from build123d import *

# Parameters (mm, degrees)
BOSS_EXTRU_1_DEPTH   = 3
ESQUISSE2_R          = 2.55
BOSS_EXTRU_2_DEPTH   = 3.2
CONG_1_R             = 1.8
D_GAGEMENT_M31_D     = 3.4
D_GAGEMENT_M31_DEPTH = 5
D_GAGEMENT_M31_TIP   = 1.021463052


with BuildPart() as part:
    # Esquisse1 → Boss.-Extru.1 (new body)
    with BuildSketch(Plane(origin=(0, 0, 0), x_dir=(1, 0, 0), z_dir=(0, 1, 0))):
        Polygon((3.117691454, 0), (1.558845727, 2.7), (-1.558845727, 2.7), (-3.117691454, 0), (-1.558845727, -2.7), (1.558845727, -2.7), align=None)
    extrude(amount=BOSS_EXTRU_1_DEPTH)

    # Esquisse2 → Boss.-Extru.2 (add)
    with BuildSketch(Plane(origin=(0, 3, 0), x_dir=(1, 0, 0), z_dir=(0, 1, 0))):
        with Locations(Location((0, 0, 0), (0, 0, 270))):
            Circle(ESQUISSE2_R)
    extrude(amount=BOSS_EXTRU_2_DEPTH)

    # Congé1
    cong_1_edges = [part.edges().sort_by_distance(p)[0] for p in [
        (0, 6.2, -2.55),
    ]]
    fillet(cong_1_edges, radius=CONG_1_R)

    # Dégagement M31
    with Locations(Plane(origin=(0, 0, 0), x_dir=(-1, 0, 0), z_dir=(0, -1, 0))):
        with Locations((0, 0)):
            Hole(D_GAGEMENT_M31_D / 2, depth=D_GAGEMENT_M31_DEPTH)
            with Locations((0, 0, -(D_GAGEMENT_M31_DEPTH + D_GAGEMENT_M31_TIP / 2))):  # 118° drill point
                Cone(0, D_GAGEMENT_M31_D / 2, D_GAGEMENT_M31_TIP, mode=Mode.SUBTRACT)


solid = part.part
Geometry check sheet. Reference: the model listing, model coordinates, mm. A direction names the side the tool comes from. Coordinates: 2 decimals unless noted, no trailing zeros. Loops run counter-clockwise (first coordinate to the right, second up) from the corner with the lowest first, then second, coordinate; pieces in that order, holes last. Notation, with made-up numbers: (43.5, -13.75) - (83.5, -13.75) arc R22 ccw to (83.5, -7.75) - close; hole circle Ø11 at (1, 45.25). An arc over 180 degrees is marked (long way). Use one line per item in the form item = value. Start each with the question number.
Item 1: Section check A-A, the plane y = 2.75. Enter the section's corners in (x, z).
Item 2: Mould release check, pull along Z, two halves, no side actions. Record for faces 1 (the face through (-0.37, 2.54, 1.66)), 2 (the face through (0, 1, 2.7)), 3 (the face through (0.064, 5.844, 0.288)), 4 (the face through (2.35, 1.48, -1.33)): +Z half, -Z half, draft (parallel to the pull), parting line (faces both ways), or undercut.
Item 3: Gauge pin test, flat ends, axial feed: pin 1 (1 mm diameter, centred on x = 1, z = -1.5, fed in from +Y); pin 2 (1 mm diameter, centred on y = 4.5, z = 1.5, fed in from -X); pin 3 (2 mm diameter, centred on x = 2, z = -2, fed in from +Y). Record the tip position at first contact, or that the pin passes through.
Item 4: Tool access check on faces 5 (the face through (-2.35, 1.48, 1.33)), 6 (the face through (0.77, 3.69, 2.43)). Record the directions out of +Z, -Z, +X, -X, +Y, -Y that give a thin tool (end or side, any length) a straight path to the whole face; none if there is none.
Item 5: Thickness scan on probe 1 along Z at (x, y) = (0, 1.5); probe 2 along Y at (x, z) = (-2.5, -0.65); probe 3 along Z at (x, y) = (1, 1.5). Record the ranges inside material, lowest first.
Computed:
q1.outline = (-3.12, 0) - (-1.56, -2.7) - (1.56, -2.7) - (3.12, 0) - (1.56, 2.7) - (-1.56, 2.7) - close; hole circle Ø3.4 at (0, 0)
q2.face_1 = undercut
q2.face_2 = +Z half
q2.face_3 = undercut
q2.face_4 = -Z half
q3.pin_1 = 6.11
q3.pin_2 = -2.34
q3.pin_3 = 5.84
q4.face_5 = +Z, -X, +Y, -Y
q4.face_6 = +Y
q5.probe_1 = -2.7 to -1.7, 1.7 to 2.7
q5.probe_2 = 0 to 3
q5.probe_3 = -2.7 to -1.37, 1.37 to 2.7
